Read the model definition and answer for the solid it produces. Units are mm, in the model's axes. Coordinates: 2 decimals unless noted, no trailing zeros. Answer in a Markdown table with one row per item.
from build123d import *

# Parameters (mm, degrees)
SKETCH_1_R      = 2
EXTRUDE_1_DEPTH = 1


with BuildPart() as part:
    # 草图1 → 凸台-拉伸1 (new body)
    with BuildSketch(Plane.XZ.offset(17.798874667)):
        with BuildLine():
            Line((-395.706204946, -91.903738718), (-395.706204946, -160.757312284))
            ThreePointArc((-395.706204946, -160.757312284), (-395.630097027, -161.139937827), (-395.413356336, -161.464311369))
            Line((-395.413356336, -161.464311369), (-386.224002242, -170.653665463))
            ThreePointArc((-386.224002242, -170.653665463), (-385.8996287, -170.870406154), (-385.517003157, -170.946514073))
            Line((-385.517003157, -170.946514073), (-326.663429591, -170.946514073))
            ThreePointArc((-326.663429591, -170.946514073), (-326.280804048, -170.870406154), (-325.956430506, -170.653665463))
            Line((-325.956430506, -170.653665463), (-316.767076412, -161.464311369))
            ThreePointArc((-316.767076412, -161.464311369), (-316.550335721, -161.139937827), (-316.474227802, -160.757312284))
            Line((-316.474227802, -160.757312284), (-316.474227802, -91.903738718))
            ThreePointArc((-316.474227802, -91.903738718), (-316.550335721, -91.521113175), (-316.767076412, -91.196739633))
            Line((-316.767076412, -91.196739633), (-325.956430506, -82.007385539))
            ThreePointArc((-325.956430506, -82.007385539), (-326.280804048, -81.790644848), (-326.663429591, -81.714536929))
            Line((-326.663429591, -81.714536929), (-385.517003157, -81.714536929))
            ThreePointArc((-385.517003157, -81.714536929), (-385.8996287, -81.790644848), (-386.224002242, -82.007385539))
            Line((-386.224002242, -82.007385539), (-395.413356336, -91.196739633))
            ThreePointArc((-395.413356336, -91.196739633), (-395.630097027, -91.521113175), (-395.706204946, -91.903738718))
        make_face()
        with Locations(Location((-388.090216374, -90.330525501, 0), (0, 0, 270))):
            Circle(SKETCH_1_R, mode=Mode.SUBTRACT)
        with Locations(Location((-324.090216374, -90.330525501, 0), (0, 0, 270))):
            Circle(SKETCH_1_R, mode=Mode.SUBTRACT)
        with Locations(Location((-324.090216374, -162.330525501, 0), (0, 0, 270))):
            Circle(SKETCH_1_R, mode=Mode.SUBTRACT)
        with Locations(Location((-388.090216374, -162.330525501, 0), (0, 0, 270))):
            Circle(SKETCH_1_R, mode=Mode.SUBTRACT)
        with BuildLine():
            add(Edge.make_bspline(
                [(-328.115549043, -154.074705918), (-328.521110277, -154.59950882), (-328.935951097, -155.116186146), (-329.806169809, -156.114044907), (-330.260453195, -156.596991611), (-331.213350311, -157.520739064), (-331.707900164, -157.955834459), (-332.723346196, -158.787049549), (-333.244315955, -159.183060394), (-334.848936349, -160.309387169), (-335.972388004, -160.980823062), (-337.731348119, -161.87882583), (-338.332266211, -162.161075436), (-339.54151706, -162.683417257), (-340.150623092, -162.924120409), (-343.216470166, -164.034826977), (-345.733148117, -164.631034044), (-349.574949627, -165.220267596), (-350.866884926, -165.364900576), (-353.472874642, -165.553124722), (-354.790025345, -165.596406642), (-358.712924122, -165.592375715), (-361.308871291, -165.414172312), (-365.167942823, -164.830251401), (-366.448430665, -164.582286392), (-368.358111819, -164.109940734), (-368.99453183, -163.935229374), (-370.254220123, -163.552000312), (-370.876741702, -163.343828387), (-372.721697987, -162.668191611), (-373.921848978, -162.150340028), (-375.669495279, -161.254671187), (-376.243225263, -160.936174353), (-377.371642786, -160.256122939), (-377.926429949, -159.894182142), (-378.998067992, -159.136743168), (-379.517159279, -158.739902065), (-380.523601029, -157.91183415), (-381.01071538, -157.480351552), (-381.943283382, -156.572254171), (-382.389831683, -156.096825252), (-383.249518774, -155.109773972), (-383.661413356, -154.596803725), (-384.064883145, -154.074706668)],
                knots=[0, 0, 0, 0, 0.03125, 0.03125, 0.0625, 0.0625, 0.09375, 0.09375, 0.125, 0.125, 0.1875, 0.1875, 0.21875, 0.21875, 0.25, 0.25, 0.375, 0.375, 0.4375, 0.4375, 0.5, 0.5, 0.625, 0.625, 0.6875, 0.6875, 0.71875, 0.71875, 0.75, 0.75, 0.8125, 0.8125, 0.84375, 0.84375, 0.875, 0.875, 0.90625, 0.90625, 0.9375, 0.9375, 0.96875, 0.96875, 1, 1, 1, 1], degree=3))
            add(Edge.make_bspline(
                [(-384.064883145, -154.074706668), (-384.765407707, -153.0864132), (-385.42732094, -152.076153161), (-386.292484546, -150.488109085), (-386.559459675, -149.946579027), (-387.059276771, -148.844100038), (-387.291729743, -148.282508818), (-388.359546252, -145.46132493), (-388.939276666, -143.138851633), (-389.482665418, -139.577278966), (-389.611388551, -138.374314162), (-389.781266573, -135.965239718), (-389.822006502, -134.76010621), (-389.851460561, -132.349137318), (-389.839404608, -131.143291545), (-389.811274153, -128.731545786), (-389.79638992, -127.525661857), (-389.796563394, -125.114297943), (-389.811529784, -123.908816727), (-389.839623007, -121.497829476), (-389.851459361, -120.292359943), (-389.821592912, -117.886702654), (-389.780638177, -116.686362914), (-389.611853133, -114.293992905), (-389.484842639, -113.101884222), (-389.123813463, -110.727901972), (-388.888904034, -109.546113603), (-388.436003689, -107.783047131), (-388.268720755, -107.197789125), (-387.904764869, -106.045116113), (-387.707679153, -105.475910785), (-387.281297017, -104.352704238), (-387.051446913, -103.79896437), (-386.556282004, -102.708224696), (-386.291397985, -102.171021551), (-385.430552687, -100.590656677), (-384.768336475, -99.578768629), (-384.064883703, -98.58634508)],
                knots=[0, 0, 0, 0, 0.0625, 0.0625, 0.09375, 0.09375, 0.125, 0.125, 0.25, 0.25, 0.3125, 0.3125, 0.375, 0.375, 0.4375, 0.4375, 0.5, 0.5, 0.5625, 0.5625, 0.625, 0.625, 0.6875, 0.6875, 0.75, 0.75, 0.8125, 0.8125, 0.84375, 0.84375, 0.875, 0.875, 0.90625, 0.90625, 0.9375, 0.9375, 1, 1, 1, 1], degree=3))
            add(Edge.make_bspline(
                [(-384.064883703, -98.58634508), (-383.659322468, -98.061542177), (-383.244481649, -97.544864852), (-382.374262935, -96.547006091), (-381.91997955, -96.064059387), (-380.967082434, -95.140311933), (-380.47253258, -94.705216539), (-379.457086548, -93.874001449), (-378.93611679, -93.477990604), (-377.331496396, -92.35166383), (-376.208044739, -91.680227937), (-374.449084625, -90.782225169), (-373.848166533, -90.499975563), (-372.638915684, -89.977633743), (-372.029809651, -89.73693059), (-368.963962577, -88.626224023), (-366.447284626, -88.030016957), (-362.605483116, -87.440783404), (-361.313547818, -87.296150424), (-358.707558102, -87.107926278), (-357.390407398, -87.064644358), (-353.467508621, -87.068675286), (-350.871561452, -87.24687869), (-347.01248992, -87.830799602), (-345.732002079, -88.078764611), (-343.822320925, -88.55111027), (-343.185900913, -88.72582163), (-341.92621262, -89.109050692), (-341.303691042, -89.317222617), (-339.458734756, -89.992859393), (-338.258583765, -90.510710976), (-336.510937465, -91.406379817), (-335.937207481, -91.724876651), (-334.808789958, -92.404928066), (-334.254002795, -92.766868862), (-333.182364752, -93.524307837), (-332.663273465, -93.92114894), (-331.656831716, -94.749216855), (-331.169717364, -95.180699453), (-330.237149362, -96.088796835), (-329.790601062, -96.564225753), (-328.930913971, -97.551277033), (-328.519019389, -98.064247281), (-328.1155496, -98.586344338)],
                knots=[0, 0, 0, 0, 0.03125, 0.03125, 0.0625, 0.0625, 0.09375, 0.09375, 0.125, 0.125, 0.1875, 0.1875, 0.21875, 0.21875, 0.25, 0.25, 0.375, 0.375, 0.4375, 0.4375, 0.5, 0.5, 0.625, 0.625, 0.6875, 0.6875, 0.71875, 0.71875, 0.75, 0.75, 0.8125, 0.8125, 0.84375, 0.84375, 0.875, 0.875, 0.90625, 0.90625, 0.9375, 0.9375, 0.96875, 0.96875, 1, 1, 1, 1], degree=3))
            add(Edge.make_bspline(
                [(-328.1155496, -98.586344338), (-327.415025038, -99.574637805), (-326.753111806, -100.584897844), (-325.8879482, -102.17294192), (-325.620973071, -102.714471978), (-325.121155975, -103.816950967), (-324.888703004, -104.378542187), (-323.820886495, -107.199726075), (-323.241156082, -109.522199372), (-322.69776733, -113.083772038), (-322.569044197, -114.286736841), (-322.399166175, -116.695811285), (-322.358426246, -117.900944793), (-322.328972188, -120.311913685), (-322.341028142, -121.517759457), (-322.369158597, -123.929505216), (-322.38404283, -125.135389145), (-322.383869357, -127.546753058), (-322.368902966, -128.752234275), (-322.340809743, -131.163221525), (-322.328973388, -132.368691057), (-322.358839836, -134.774348346), (-322.399794572, -135.974688086), (-322.568579615, -138.367058095), (-322.695590109, -139.559166777), (-323.056619285, -141.933149027), (-323.291528714, -143.114937396), (-323.744429058, -144.878003867), (-323.911711993, -145.463261874), (-324.275667878, -146.615934885), (-324.472753594, -147.185140214), (-324.899135729, -148.30834676), (-325.128985833, -148.862086628), (-325.624150742, -149.952826302), (-325.889034762, -150.490029447), (-326.74988006, -152.07039432), (-327.412096271, -153.082282368), (-328.115549043, -154.074705918)],
                knots=[0, 0, 0, 0, 0.0625, 0.0625, 0.09375, 0.09375, 0.125, 0.125, 0.25, 0.25, 0.3125, 0.3125, 0.375, 0.375, 0.4375, 0.4375, 0.5, 0.5, 0.5625, 0.5625, 0.625, 0.625, 0.6875, 0.6875, 0.75, 0.75, 0.8125, 0.8125, 0.84375, 0.84375, 0.875, 0.875, 0.90625, 0.90625, 0.9375, 0.9375, 1, 1, 1, 1], degree=3))
        make_face(mode=Mode.SUBTRACT)
    extrude(amount=EXTRUDE_1_DEPTH)


solid = part.part
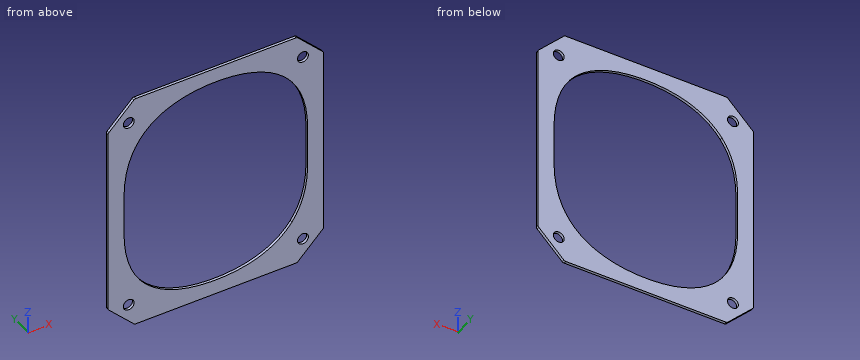
Q1. Consider line 1 (X direction, y = -18.65, z = -119); line 2 (Z direction, x = -325, y = -18.7); line 3 (X direction, y = -18.7, z = -105.5). Determine where each line is inside the solid, lowest interval first.
Outcome:
| item | result |
|---|---|
| line 1 | -395.71 to -389.84, -322.35 to -316.47 |
| line 2 | -169.7 to -164.11, -160.55 to -148.54, -104.12 to -92.11, -88.55 to -82.96 |
| line 3 | -395.71 to -387.71, -324.47 to -316.47 |
Q2. Given pin 1 (3 mm diameter, centred on x = -324.09, z = -90.33, fed in from -Y), flat-ended and moving along its own axis, determine where the tip first touches the part or whether it passes through.
Outcome:
| item | result |
|---|---|
| pin 1 | through |
Q3. The part is cut by section A-A (z = -90). Give the number of separate pieces and of enclosed holes in the cut face, then the cut area to 3 significant figures.
Outcome:
| item | result |
|---|---|
| separate pieces | 4 |
| enclosed holes | 0 |
| area | 35.2 mm² |
